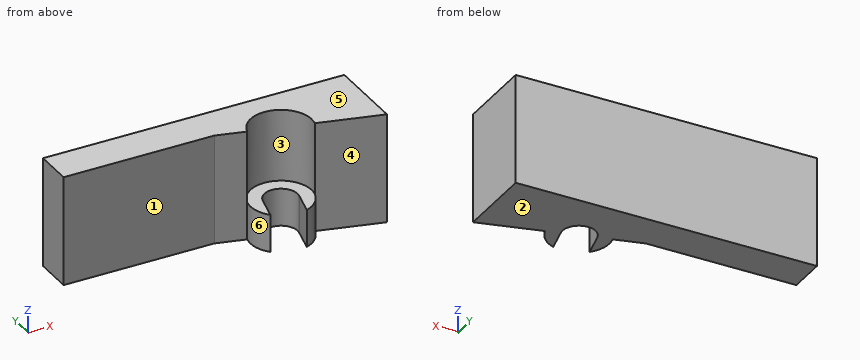
```python
from build123d import *

# Parameters (mm, degrees)
F1_DEPTH  = 25.4
F3_DEPTH  = 152.4
F4_R      = 5.1395
F5_DEPTH  = 152.401
F7_DEPTH  = 6.096
F9_DEPTH  = 6.35
F10_R     = 1.905
F11_DEPTH = 6.35
F12_W     = 46.7241909355
F12_H     = 189.791161567
F13_DEPTH = 50.801


with BuildPart() as f1:
    # F0 (on Right) → F1 (new body)
    with BuildSketch(Plane.YZ):
        Polygon((-6.35, 0), (0, 0), (0, 203.2), (-24.13, 203.2), (-24.13, 177.8), (-17.78, 177.8), (-17.78, 196.85), (-6.35, 196.85), align=None)
    extrude(amount=F1_DEPTH)

    # F2 (on Top) → F3 (join)
    with BuildSketch(Plane.XY):
        Polygon((50.8, 0), (25.4, 0), (25.4, -6.35), (50.8, -13.1559094878), align=None)
    extrude(amount=F3_DEPTH)

    # F4 (on face) → F5 (cut, through all)
    with BuildSketch(Plane.XY.offset(152.4)):
        with Locations((35.2138063951, -8.9796014982)):
            Circle(F4_R)
    extrude(amount=-F5_DEPTH, mode=Mode.SUBTRACT)

    # F6 (on face) → F7 (cut)
    with BuildSketch(Plane.YZ.offset(50.8)):
        Polygon((-9.3719547439, 71.3606500437), (-3.7839547439, 71.3606500437), (-0.9899547439, 76.2), (-3.7839547439, 81.0393499563), (-9.3719547439, 81.0393499563), (-12.1659547439, 76.2), align=None)
    extrude(amount=-F7_DEPTH, mode=Mode.SUBTRACT)

    # F8 (on face) → F9 (join)
    with BuildSketch(Plane(origin=(0, 0, 0), x_dir=(1, 0, 0), z_dir=(0, 0, -1))):
        with BuildLine():
            Line((32.4918402484, 8.3672288206), (31.4877265179, 12.5194869482))
            ThreePointArc((31.4877265179, 12.5194869482), (30.2327985505, 10.2461010452), (30.2494306109, 7.6494010159))
            ThreePointArc((30.2494306109, 7.6494010159), (36.5440068774, 4.015225714), (40.1781821793, 10.3098019805))
            ThreePointArc((40.1781821793, 10.3098019805), (38.9811201217, 12.4755716834), (36.9107028801, 13.8308902517))
            Line((36.9107028801, 13.8308902517), (37.9148166106, 9.678632124))
            ThreePointArc((37.9148166106, 9.678632124), (37.9256407477, 9.6353868624), (37.9357725418, 9.5919741759))
            ThreePointArc((37.9357725418, 9.5919741759), (35.8261790728, 6.2576353516), (32.4918402484, 8.3672288206))
        make_face()
    extrude(amount=-F9_DEPTH)

    # F10 (on face) → F11 (join)
    with BuildSketch(Plane(origin=(0.1139773719, 0.425369343, 0), x_dir=(0.9659258263, -0.2588190451, 0), z_dir=(-0.2588190451, -0.9659258263, 0))):
        with Locations((45.3620319066, 149.352)):
            Circle(F10_R)
        with Locations((49.4260319066, 145.288)):
            Circle(F10_R)
    extrude(amount=F11_DEPTH)

    # F12 (on face) → F13 (cut, through all)
    with BuildSketch(Plane.YZ.offset(50.8)):
        with Locations((-7.7233714983, 113.3844163269)):
            Rectangle(F12_W, F12_H)
    extrude(amount=-F13_DEPTH, mode=Mode.SUBTRACT)


solid = f1.part
```
Work out the finished part from the listing and answer in its coordinate system (mm). Face numbers are marked on the shaded views. A direction names the side the tool comes from. Give positions to 0.01 mm unless a question says otherwise; leave off trailing zeros. Order: outer loops, then holes, each group sorted by start corner. A loop starts at its lowest first (then second) coordinate and runs counter-clockwise, first axis right, second up.
1. The mould has two halves that part along X. Classify the marked faces 4, 5 and 6: released by +X, released by -X, zero draft, split by the parting line, or undercut.
Result sheet:
face 4: undercut
face 5: zero draft
face 6: released by -X
2. Section C-C, the plane x = 38.5 is taken. Determine the outline of the cut face in (y, z).
Result sheet:
outline: (-12.93, 0) - (0, 0) - (0, 18.49) - (-5.03, 18.49) - (-5.03, 6.35) - (-12.93, 6.35) - close
3. For the marked faces 1, 2 and 3, determine the directions among +Z, -Z, +X, -X, +Y, -Y from which every point of the face is accessible in a straight line to the end or side of a thin tool.
Result sheet:
face 1: +Z, -Z, -X, -Y
face 2: -Z, +X, -X, +Y, -Y
face 3: +Z
4. Straight lines are drawn through the part: L1, parallel to Y at x = 15.5, z = 14; L2, parallel to Z at x = 37.5, y = -5.5; L3, parallel to Y at x = 35, z = 2.5. For each, find the intervals that lie inside material, in ascending order.
Result sheet:
L1: y = -6.35 to 0
L2: z = 0 to 6.35
L3: y = -6.2 to 0
5. Section B-B, the plane y = -11.5 is taken. Determine the outline of the cut face in (x, z).
Result sheet:
outline: (30.73, 0) - (31.73, 0) - (31.73, 6.35) - (30.73, 6.35) - close; (37.47, 0) - (39.69, 0) - (39.69, 6.35) - (37.47, 6.35) - close; (44.62, 0) - (50.8, 0) - (50.8, 18.49) - (44.62, 18.49) - close
6. Section A-A, the plane z = 8.5 is taken. Determine the outline of the cut face in (x, y).
Result sheet:
outline: (0, -6.35) - (25.4, -6.35) - (30.25, -7.65) arc R5.14 cw to (40.18, -10.31) - (50.8, -13.16) - (50.8, 0) - (0, 0) - close
7. Each of these flat-tipped pins is pushed along its axis until it touches: P1, Ø8, axis at x = 17, z = 2, coming from the +Y side; P2, Ø3, axis at x = 14.5, z = 7.5, coming from the -Y side. Where does it stop, or does it pass through?
Result sheet:
P1: stops at y = 0
P2: stops at y = -6.35
8. Section D-D, the plane y = -5.5 is taken. Determine the outline of the cut face in (x, z).
Result sheet:
outline: (0, 0) - (50.8, 0) - (50.8, 18.49) - (39, 18.49) - (39, 6.35) - (31.43, 6.35) - (31.43, 18.49) - (0, 18.49) - close
